Could you check a few things on this drawing? It's one solid part, dimensions in mm from its lowest x, y, z. A direction names the side the tool comes from. Give positions to 0.01 mm unless a question says otherwise; leave off trailing zeros. Order: outer loops, then holes, each group sorted by start corner. A loop starts at its lowest first (then second) coordinate and runs counter-clockwise, first axis right, second up. Notation, with made-up numbers: (81.25, 76) -> (85.25, 76) arc R9 cw to (85.25, 91) -> close; hole circle Ø4 at (28.25, -1). An arc over 180 degrees is marked (long way). Answer as a JSON object with one key per item and string values.
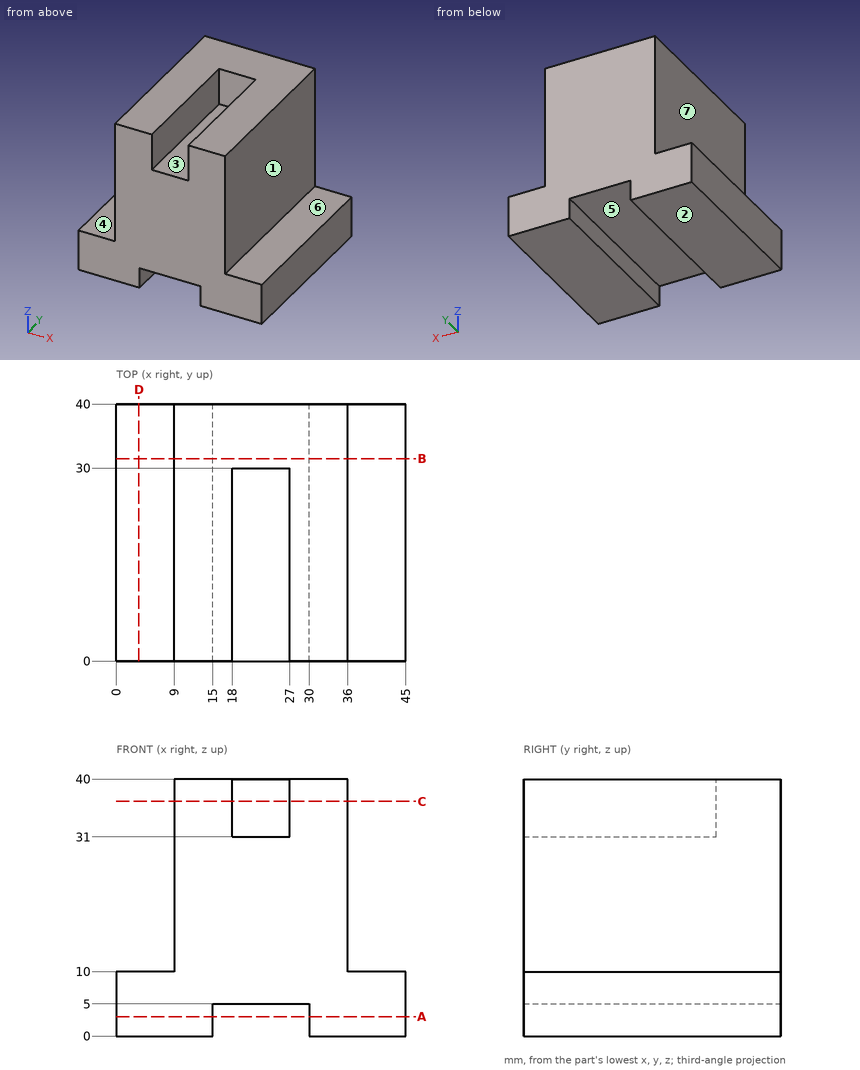
1. For the marked faces 1, 2, 3 and 4, which set-ups out of +Z, -Z, +X, -X, +Y, -Y let a thin tool reach every point of the face, with its end or its side?
Worked answers:
{"face 1": "+Z, +X, +Y, -Y", "face 2": "-Z, +X, -X, +Y, -Y", "face 3": "+Z, -Y", "face 4": "+Z, -X, +Y, -Y"}
2. If we section it at C-C on z = 36.5: Please give me the cut outline in (x, y), then the cut area to 3 significant figures.
Worked answers:
{"outline": "(9, 0) -> (18, 0) -> (18, 30) -> (27, 30) -> (27, 0) -> (36, 0) -> (36, 40) -> (9, 40) -> close", "area": "810 mm²"}
3. If we section it at D-D on x = 3.5: Please give me the cut outline in (y, z).
Worked answers:
{"outline": "(0, 0) -> (40, 0) -> (40, 10) -> (0, 10) -> close"}
4. Will these pins go through, and if not, where does the flat tip stop? pin 1 Ø24 at (y, z) = (26, 24.5) entering from +X; pin 2 Ø2.5 at (x, y) = (38.5, 10) entering from +Z; pin 3 Ø7 at (x, y) = (23, 9) entering from +Z.
Worked answers:
{"pin 1": "x = 36", "pin 2": "z = 10", "pin 3": "z = 31"}
5. If we mould it in two halves opening along X, with no side actions, what happens to the marked faces 5, 6 and 7? For each: +X half, -X half, draft (parallel to the pull), parting line (faces both ways), or undercut.
Worked answers:
{"face 5": "undercut", "face 6": "draft", "face 7": "-X half"}
6. If we section it at B-B on y = 31.5: Please give me the cut outline in (x, z), then the cut area to 4 significant figures.
Worked answers:
{"outline": "(0, 0) -> (15, 0) -> (15, 5) -> (30, 5) -> (30, 0) -> (45, 0) -> (45, 10) -> (36, 10) -> (36, 40) -> (9, 40) -> (9, 10) -> (0, 10) -> close", "area": "1,185 mm²"}
7. Please list where these lines run through material, in increasing order: L1, parallel to Z at x = 22, y = 15; L2, parallel to X at y = 17, z = 17.5; L3, parallel to Z at x = 39.5, y = 33.
Worked answers:
{"L1": "5 to 31", "L2": "9 to 36", "L3": "0 to 10"}
8. If we section it at A-A on z = 3: Please give me the cut outline in (x, y), then the cut area to 3 significant figures.
Worked answers:
{"outline": "(0, 0) -> (15, 0) -> (15, 40) -> (0, 40) -> close; (30, 0) -> (45, 0) -> (45, 40) -> (30, 40) -> close", "area": "1,200 mm²"}
